For this review, take the finished solid that the model builds, in its own axes (mm). Coordinates: 2 decimals unless noted, no trailing zeros. Loops run counter-clockwise (first coordinate to the right, second up) from the corner with the lowest first, then second, coordinate; pieces in that order, holes last. Notation, with made-up numbers: (39.25, 39) -> (46.25, 39) arc R28 cw to (46.25, 70) -> close; hole circle Ø5 at (56, 62.25). An arc over 180 degrees is marked (long way). Answer in a Markdown table with one row per item.
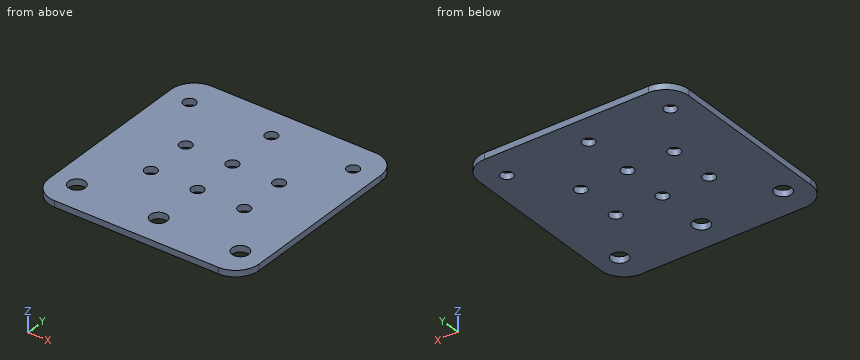
Autodesk Inventor part; units mm, degrees
ref_plane "YZ Plane" through (0, 0, 0) normal (1, 0, 0) x (0, 1, 0)
ref_plane "XZ Plane" through (0, 0, 0) normal (0, 1, 0) x (-1, 0, 0)
ref_plane "XY Plane" through (0, 0, 0) normal (0, 0, 1) x (1, 0, 0)
sketch "Sketch1" plane through (0, 0, 0) normal (0, 0, 1) x (1, 0, 0)
  line L0 (-45, 45) -> (45, 45)
  line L1 (45, 45) -> (45, -45)
  line L2 (45, -45) -> (-45, -45)
  line L3 (-45, -45) -> (-45, 45)
  point P0 (0, 0)
  dimension "d0" = 90
  dimension "d1" = 90
  dimension "d2" = 45
  dimension "d3" = 45
extrude "Extrusion1" add sketch "Sketch1" along normal blind 2.6568
fillet "Fillet1" radius 10 4 edges at (45, 45, 1.3284) (-45, 45, 1.3284) (45, -45, 1.3284) (-45, -45, 1.3284)
sketch "Sketch2" plane through (0, 0, 2.6568) normal (0, 0, 1) x (1, 0, 0)
  line L0 (45, 35) -> (45, -35)
  line L1 (-35, 45) -> (35, 45)
  circle A0 centre (35, 32.3) radius 2.6
  circle A1 centre (35, -32.3) radius 3.5685
  point P0 (0, 0)
  dimension "d7" = 5.2
  dimension "d8" = 10
  dimension "d10" = 7.137
  dimension "d12" = 10
  dimension "d52" = 64.6
  dimension "d53" = 12.7
extrude "Extrusion2" cut sketch "Sketch2" against normal through all
pattern_linear "Rectangular Pattern1" count 3 spacing 35 along (-1, 0, 0) of "Extrusion2"
sketch "Sketch3" plane through (0, 0, 2.6568) normal (0, 0, 1) x (1, 0, 0)
  line L0 (35, -45) -> (-35, -45)
  line L1 (-45, -35) -> (-45, 35)
  circle A0 centre (-20, -10) radius 2.6
  point P0 (0, 0)
  dimension "d18" = 5.2
  dimension "d19" = 25
  dimension "d20" = 35
extrude "Extrusion3" cut sketch "Sketch3" against normal through all
pattern_linear "Rectangular Pattern2" count 3 spacing 20 along (1, 0, 0) count 2 spacing 20 along (0, 1, 0) of "Extrusion3"
properties part number "spindle_mount_plate" material "Steel, Mild"
Item 1: Take a section at C-C, the plane z = 1.25. Count the separate pieces of the cut face and the enclosed holes in it, and give its area (3 significant figures).
Worked answers:
| item | result |
|---|---|
| separate pieces | 1 |
| enclosed holes | 12 |
| area | 7,700 mm² |
Item 2: For L1, parallel to Y at x = 20, z = 2; L2, parallel to Y at x = 35, z = 0.75; L3, parallel to X at y = -33, z = 0.2, list the stretches that pass through material, from the lowest coordinate up.
Worked answers:
| item | result |
|---|---|
| L1 | -45 to -12.6, -7.4 to 7.4, 12.6 to 45 |
| L2 | -45 to -35.87, -28.73 to 29.7, 34.9 to 45 |
| L3 | -45 to -38.5, -31.5 to -3.5, 3.5 to 31.5, 38.5 to 45 |
Item 3: Take a section at B-B, the plane x = 0. State the section outline as (y, z) points, and give its area (3 significant figures).
Worked answers:
| item | result |
|---|---|
| outline | (-45, 0) -> (-35.87, 0) -> (-35.87, 2.66) -> (-45, 2.66) -> close; (-28.73, 0) -> (-12.6, 0) -> (-12.6, 2.66) -> (-28.73, 2.66) -> close; (-7.4, 0) -> (7.4, 0) -> (7.4, 2.66) -> (-7.4, 2.66) -> close; (12.6, 0) -> (29.7, 0) -> (29.7, 2.66) -> (12.6, 2.66) -> close; (34.9, 0) -> (45, 0) -> (45, 2.66) -> (34.9, 2.66) -> close |
| area | 179 mm² |
Item 4: Take a section at A-A, the plane y = 10. State the section outline as (x, z) points.
Worked answers:
| item | result |
|---|---|
| outline | (-45, 0) -> (-22.6, 0) -> (-22.6, 2.66) -> (-45, 2.66) -> close; (-17.4, 0) -> (-2.6, 0) -> (-2.6, 2.66) -> (-17.4, 2.66) -> close; (2.6, 0) -> (17.4, 0) -> (17.4, 2.66) -> (2.6, 2.66) -> close; (22.6, 0) -> (45, 0) -> (45, 2.66) -> (22.6, 2.66) -> close |
Item 5: Insertion check: pin 1 (1.5 mm diameter, centred on x = 27, y = -17, fed in from -Z). The pin has a flat end and moves straight along its axis. Give the tip position at first contact, or say it passes through.
Worked answers:
| item | result |
|---|---|
| pin 1 | z = 0 |
Item 6: Take a section at D-D, the plane x = -36.5. State the section outline as (y, z) points.
Worked answers:
| item | result |
|---|---|
| outline | (-44.89, 0) -> (-35.54, 0) -> (-35.54, 2.66) -> (-44.89, 2.66) -> close; (-29.06, 0) -> (30.18, 0) -> (30.18, 2.66) -> (-29.06, 2.66) -> close; (34.42, 0) -> (44.89, 0) -> (44.89, 2.66) -> (34.42, 2.66) -> close |
